```python
from build123d import *

# Parameters (mm, degrees)
SKETCH_1_W      = 300
SKETCH_1_H      = 300
EXTRUDE_1_DEPTH = 90
SKETCH_2_W      = 20
SKETCH_2_H      = 300
SKETCH_2_W_2    = 300
SKETCH_2_H_2    = 20
EXTRUDE_3_DEPTH = 10
SKETCH_6_W      = 140
SKETCH_6_H      = 140
EXTRUDE_6_DEPTH = 9


with BuildPart() as part:
    # Эскиз1 → Бобышка-Вытянуть1 (new body)
    with BuildSketch(Plane(origin=(0, 0, 0), x_dir=(1, 0, 0), z_dir=(0, 1, 0))):
        Rectangle(SKETCH_1_W, SKETCH_1_H)
    extrude(amount=EXTRUDE_1_DEPTH)

    # Эскиз2 → Бобышка-Вытянуть3 (add)
    with BuildSketch(Plane(origin=(0, 90, 0), x_dir=(1, 0, 0), z_dir=(0, 1, 0))):
        Rectangle(SKETCH_2_W, SKETCH_2_H)
        Rectangle(SKETCH_2_W_2, SKETCH_2_H_2)
    extrude(amount=EXTRUDE_3_DEPTH)

    # Эскиз6 → Бобышка-Вытянуть6 (add)
    with BuildSketch(Plane(origin=(0, 90, 0), x_dir=(1, 0, 0), z_dir=(0, 1, 0))):
        with Locations((-80, -80)):
            Rectangle(SKETCH_6_W, SKETCH_6_H)
        with Locations((80, -80)):
            Rectangle(SKETCH_6_W, SKETCH_6_H)
        with Locations((80, 80)):
            Rectangle(SKETCH_6_W, SKETCH_6_H)
        with Locations((-80, 80)):
            Rectangle(SKETCH_6_W, SKETCH_6_H)
    extrude(amount=EXTRUDE_6_DEPTH)


solid = part.part
```
The listing builds one solid part. Answer for the finished solid, in the listing's coordinates (mm). A direction names the side the tool comes from. Coordinates: 2 decimals unless noted, no trailing zeros. Answer as a JSON object with one key per item and string values. Group by question number.
1. A straight line is drawn through the part: line 1 (Y direction, x = -134.5, z = -108.5). Find the intervals that lie inside material, in ascending order.
2. A tool of negligible diameter and unlimited length cuts with its end or side. For faces 1 (the flat face through (79, 99, -81)), 2 (the flat face through (-81, 99, -81)), 3 (the flat face through (79, 99, 79)), from which of +Z, -Z, +X, -X, +Y, -Y can it reach the whole face along a straight path? Write none if from no direction.
3. Flat-ended cylindrical pins translate along their axes: P1, Ø0.8, axis at y = 99.5, z = 81, coming from the +X side; P2, Ø0.8, axis at x = 73, y = 99.5, coming from the -Z side; P3, Ø1.5, axis at x = 15.5, z = 72.5, coming from the -Y side; P4, Ø0.5, axis at y = 99.5, z = -66, coming from the -X side. Find the tip coordinate at first contact, or state that the pin passes through.
Values follow:
{
 "1": {"line 1": "0 to 99"},
 "2": {"face 1": "-Z, +X, +Y", "face 2": "-Z, -X, +Y", "face 3": "+Z, +X, +Y"},
 "3": {"P1": "x = 10", "P2": "z = -10", "P3": "y = 0", "P4": "x = -10"}
}
